Source: CAD feature listing. Evaluate the final solid. Frame: model axes, mm. Coordinates: 2 decimals unless noted, no trailing zeros. Loops run counter-clockwise (first coordinate to the right, second up) from the corner with the lowest first, then second, coordinate; pieces in that order, holes last.
Item 1: Section query A-A, the plane z = 40. Return the cut outline in (x, y), then the cut area to 3 significant figures.
Item 2: Line query: probe 1 along Z at (x, y) = (3.5, 0.5); probe 2 along X at (y, z) = (2.65, 22.5); probe 3 along X at (y, z) = (1.75, -40). Output: solid intervals per line, ascending.
Item 3: Section query C-C, the plane x = 77.5. Return the cut outline in (y, z), then the cut area to 3 significant figures.
Item 4: Section query B-B, the plane z = -22. Return the cut outline in (x, y).
Item 5: Pin query (flat end, axial travel): pin 1 Ø1.5 at (y, z) = (1, -31.5) entering from -X; pin 2 Ø2.5 at (x, z) = (24.5, 29) entering from +Y; pin 3 Ø1.5 at (x, y) = (45, 1.5) entering from -Z. Return the tip coordinate at first contact, or that it passes through.
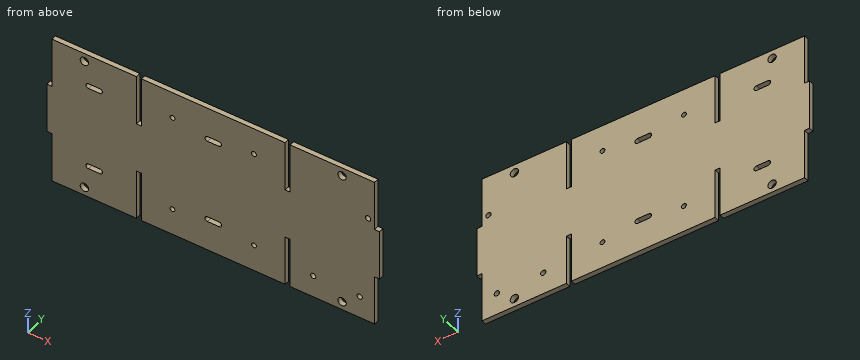
```python
from build123d import *

# Parameters (mm, degrees)
SKETCH1_W           = 200
SKETCH1_H           = 90
BOSS_EXTRUDE1_DEPTH = 3
SKETCH2_W           = 3
SKETCH2_H           = 30
CUT_EXTRUDE1_DEPTH  = 110.69958979
SKETCH3_W           = 3
SKETCH3_H           = 30
CUT_EXTRUDE2_DEPTH  = 110.69958979
SKETCH4_R           = 1.45
SKETCH4_R_2         = 1.5875
SKETCH4_W           = 10
SKETCH4_H           = 3
CUT_EXTRUDE3_DEPTH  = 110.69958979
FILLET1_R           = 1.5
SKETCH5_R           = 2.5
CUT_EXTRUDE4_DEPTH  = 110.69958979


with BuildPart() as part:
    # Sketch1 → Boss-Extrude1 (new body)
    with BuildSketch(Plane(origin=(0, 0, 0), x_dir=(1, 0, 0), z_dir=(0, 1, 0))):
        Rectangle(SKETCH1_W, SKETCH1_H)
    extrude(amount=BOSS_EXTRUDE1_DEPTH)

    # Sketch2 → Cut-Extrude1 (cut, through all)
    with BuildSketch(Plane(origin=(0, 3, 0), x_dir=(1, 0, 0), z_dir=(0, 1, 0))):
        with Locations((-98.5, 30)):
            Rectangle(SKETCH2_W, SKETCH2_H)
        with Locations((-98.5, -30)):
            Rectangle(SKETCH2_W, SKETCH2_H)
    cut_extrude1 = extrude(amount=-CUT_EXTRUDE1_DEPTH, mode=Mode.SUBTRACT)

    # Mirror1: Cut-Extrude1 across plane
    add(cut_extrude1.mirror(Plane(origin=(0, 0, 0), x_dir=(0, 0, 1), z_dir=(1, 0, 0))), mode=Mode.SUBTRACT)

    # Sketch3 → Cut-Extrude2 (cut, through all)
    with BuildSketch(Plane(origin=(0, 3, 0), x_dir=(1, 0, 0), z_dir=(0, 1, 0))):
        with Locations((44.7, 30)):
            Rectangle(SKETCH3_W, SKETCH3_H)
        with Locations((44.7, -30)):
            Rectangle(SKETCH3_W, SKETCH3_H)
    cut_extrude2 = extrude(amount=-CUT_EXTRUDE2_DEPTH, mode=Mode.SUBTRACT)

    # Mirror2: Cut-Extrude2 across plane
    add(cut_extrude2.mirror(Plane(origin=(0, 0, 0), x_dir=(0, 0, 1), z_dir=(1, 0, 0))), mode=Mode.SUBTRACT)

    # Sketch4 → Cut-Extrude3 (cut, through all)
    with BuildSketch(Plane.XZ):
        with Locations(Location((-24.5, 29, 0), (0, 0, 270))):
            Circle(SKETCH4_R)
        with Locations(Location((24.5, 29, 0), (0, 0, 270))):
            Circle(SKETCH4_R)
        with Locations(Location((24.5, -29, 0), (0, 0, 270))):
            Circle(SKETCH4_R)
        with Locations(Location((-24.5, -29, 0), (0, 0, 270))):
            Circle(SKETCH4_R)
        with Locations(Location((93.13, 20.32, 0), (0, 0, 270))):
            Circle(SKETCH4_R_2)
        with Locations(Location((60.11, -31.75, 0), (0, 0, 270))):
            Circle(SKETCH4_R_2)
        with Locations(Location((88.05, -31.75, 0), (0, 0, 270))):
            Circle(SKETCH4_R_2)
        with Locations((0, 25.5)):
            Rectangle(SKETCH4_W, SKETCH4_H)
        with Locations((0, -25.5)):
            Rectangle(SKETCH4_W, SKETCH4_H)
        with Locations((-71.6, 25.5)):
            Rectangle(SKETCH4_W, SKETCH4_H)
        with Locations((-71.6, -25.5)):
            Rectangle(SKETCH4_W, SKETCH4_H)
    extrude(amount=-CUT_EXTRUDE3_DEPTH, mode=Mode.SUBTRACT)

    # Fillet1
    fillet1_edges = [part.edges().sort_by_distance(p)[0] for p in [
        (-5, 1.5, -27),
        (-5, 1.5, -24),
        (5, 1.5, -24),
        (5, 1.5, -27),
        (-5, 1.5, 24),
        (-5, 1.5, 27),
        (5, 1.5, 27),
        (5, 1.5, 24),
        (-76.6, 1.5, 24),
        (-76.6, 1.5, 27),
        (-66.6, 1.5, 27),
        (-66.6, 1.5, -24),
        (-66.6, 1.5, -27),
        (-76.6, 1.5, -27),
        (-76.6, 1.5, -24),
        (-66.6, 1.5, 24),
    ]]
    fillet(fillet1_edges, radius=FILLET1_R - 0.0001)  # a hair under: the kernel refuses the full size

    # Sketch5 → Cut-Extrude4 (cut, through all)
    with BuildSketch(Plane(origin=(0, 3, 0), x_dir=(1, 0, 0), z_dir=(0, 1, 0))):
        with Locations(Location((-77.5, 40, 0), (0, 0, 270))):
            Circle(SKETCH5_R)
        with Locations(Location((77.5, 40, 0), (0, 0, 270))):
            Circle(SKETCH5_R)
        with Locations(Location((77.5, -40, 0), (0, 0, 270))):
            Circle(SKETCH5_R)
        with Locations(Location((-77.5, -40, 0), (0, 0, 270))):
            Circle(SKETCH5_R)
    extrude(amount=-CUT_EXTRUDE4_DEPTH, mode=Mode.SUBTRACT)


solid = part.part
```
Verdict:
1. outline: (-97, 0) - (-80, 0) - (-80, 3) - (-97, 3) - close; (-75, 0) - (-46.2, 0) - (-46.2, 3) - (-75, 3) - close; (-43.2, 0) - (43.2, 0) - (43.2, 3) - (-43.2, 3) - close; (46.2, 0) - (75, 0) - (75, 3) - (46.2, 3) - close; (80, 0) - (97, 0) - (97, 3) - (80, 3) - close
1. area: 534 mm2
2. probe 1: z = -45 to -27, -24 to 24, 27 to 45
2. probe 2: x = -97 to -46.2, -43.2 to 43.2, 46.2 to 97
2. probe 3: x = -97 to -80, -75 to -46.2, -43.2 to 43.2, 46.2 to 75, 80 to 97
3. outline: (0, -45) - (3, -45) - (3, -42.5) - (0, -42.5) - close; (0, -37.5) - (3, -37.5) - (3, 37.5) - (0, 37.5) - close; (0, 42.5) - (3, 42.5) - (3, 45) - (0, 45) - close
3. area: 240 mm2
4. outline: (-97, 0) - (-46.2, 0) - (-46.2, 3) - (-97, 3) - close; (-43.2, 0) - (43.2, 0) - (43.2, 3) - (-43.2, 3) - close; (46.2, 0) - (97, 0) - (97, 3) - (46.2, 3) - close
5. pin 1: stops at x = -97
5. pin 2: passes through
5. pin 3: stops at z = -15
